The listing builds one solid part. Answer for the finished solid, in the listing's coordinates (mm). A direction names the side the tool comes from. Coordinates: 2 decimals unless noted, no trailing zeros. Loops run counter-clockwise (first coordinate to the right, second up) from the corner with the lowest first, then second, coordinate; pieces in that order, holes last. Notation, with made-up numbers: M -35,-22.75 L 16,-22.75 A10 cw 16,-15.75 Z; hole C 81,40 d9. An arc over 180 degrees is marked long. Answer as a JSON object with one key per item and string values. Group by question number.
1. Straight lines are drawn through the part: L1, parallel to X at y = 13.5, z = 24; L2, parallel to X at y = 24.9, z = 12.7 (3 decimals); L3, parallel to X at y = 12.7, z = 0.8 (1 decimal). For each, find the intervals that lie inside material, in ascending order.
2. Determine the mould class of faces 3 (the face through (301, 25.4, 13)), 4 (the face through (8.684, 10.14, 0.814)), 5 (the face through (301, 13, 0)) for opening direction Y: released by +Y, released by -Y, zero draft, split by the parting line, or undercut.
3. For faces 1 (the face through (301, 23.749, 13)), 2 (the face through (8.684, 10.14, 24.563)), determine the directions among +Z, -Z, +X, -X, +Y, -Y from which every point of the face is accessible in a straight line to the end or side of a thin tool.
4. A cutting plane is placed at A-A on z = 19.75. Give the vertices of the cut face in (x, y).
5. A cutting plane is placed at B-B on x = 103.5. Give the vertices of the cut face in (y, z).
Autodesk Inventor part; units mm, degrees
ref_plane "YZ Plane" through (0, 0, 0) normal (1, 0, 0) x (0, 1, 0)
ref_plane "XZ Plane" through (0, 0, 0) normal (0, 1, 0) x (-1, 0, 0)
ref_plane "XY Plane" through (0, 0, 0) normal (0, 0, 1) x (1, 0, 0)
sketch "Sketch1" plane through (0, 0, 0) normal (1, 0, 0) x (0, 1, 0)
  line L0 (0, 0) -> (25.4, 0)
  line L1 (25.4, 0) -> (25.4, 25.4)
  line L2 (25.4, 25.4) -> (0, 25.4)
  line L3 (0, 25.4) -> (0, 0)
  line L4 (1.651, 23.749) -> (23.749, 23.749)
  line L5 (23.749, 23.749) -> (23.749, 1.651)
  line L6 (23.749, 1.651) -> (1.651, 1.651)
  line L7 (1.651, 1.651) -> (1.651, 23.749)
  dimension "d0" = 25.4
  dimension "d2" = 25.4
  dimension "d3" = 1.651
  dimension "d5" = 1.651
  dimension "d6" = 1.651
  dimension "d7" = 1.651
extrude "Extrusion1" add sketch "Sketch1" along normal blind 609.6
sketch "Sketch2" plane through (0, 0, 25.4) normal (0, 0, 1) x (1, 0, 0)
  line L0 (0, 25.4) -> (0, 0)
  line L1 (0, 25.4) -> (609.6, 25.4)
  point P0 (12.7, 12.7)
  dimension "d10" = 12.7
  dimension "d11" = 12.7
hole "Hole1" at (12.7, 12.7, 25.4) direction (0, 0, -1) diameter 9.525 end through all
sketch "Sketch3" plane through (0, 25.4, 25.4) normal (0, 1, 0) x (1, 0, 0)
  line L0 (609.6, 25.4) -> (609.6, 0)
  point P0 (590.55, 12.7)
  point P1 (552.45, 12.7)
  dimension "d19" = 19.05
  dimension "d20" = 38.1
hole "Hole2" at (590.55, 25.4, 12.7) at (552.45, 25.4, 12.7) direction (0, -1, 0) diameter 6.35 end through all
sketch "Sketch4" plane through (0, 0, 25.4) normal (0, 0, 1) x (1, 0, 0)
  line L0 (0, 25.4) -> (0, 0)
  line L1 (0, 0) -> (609.6, 0)
  line L2 (0, 25.4) -> (609.6, 25.4)
  point P0 (177.8, 12.7)
  point P1 (228.6, 12.7)
  dimension "d28" = 177.8
  dimension "d29" = 12.7
  dimension "d37" = 12.7
  dimension "d38" = 50.8
hole "Hole3" at (177.8, 12.7, 25.4) at (228.6, 12.7, 25.4) direction (0, 0, -1) diameter 6.35 end through all
properties part number "ArmBAr" material "Aluminum 6061"
From the geometry:
{
 "1": {"L1": "x = 0 to 8.01, 17.39 to 174.73, 180.87 to 225.53, 231.67 to 609.6", "L2": "x = 0 to 549.275, 555.625 to 587.375, 593.725 to 609.6", "L3": "x = 0 to 7.9, 17.5 to 174.6, 181 to 225.4, 231.8 to 609.6"},
 "2": {"face 3": "released by +Y", "face 4": "undercut", "face 5": "zero draft"},
 "3": {"face 1": "+X, -X", "face 2": "+Z, -Z"},
 "4": {"outline": "M 0,0 L 609.6,0 L 609.6,1.65 L 0,1.65 Z; M 0,23.75 L 609.6,23.75 L 609.6,25.4 L 0,25.4 Z"},
 "5": {"outline": "M 0,0 L 25.4,0 L 25.4,25.4 L 0,25.4 Z; hole M 1.65,1.65 L 23.75,1.65 L 23.75,23.75 L 1.65,23.75 Z"}
}
